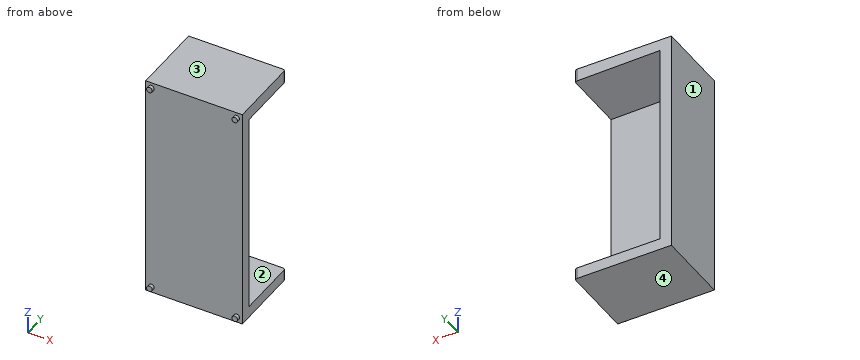
from build123d import *

# Parameters (mm, degrees)
BOSS_EXTRUDE1_DEPTH = 2000
CUT_EXTRUDE1_DEPTH  = 550
SKETCH4_R           = 25
BOSS_EXTRUDE2_DEPTH = 30


with BuildPart() as part:
    # Sketch1 → Boss-Extrude1 (new body)
    with BuildSketch(Plane.XY):
        with BuildLine():
            Line((-425, 270.9650644), (405, 270.9650644))
            ThreePointArc((405, 270.9650644), (419.142135624, 265.107200024), (425, 250.9650644))
            Line((425, 250.9650644), (425, -379.0349356))
            Line((425, -379.0349356), (-425, -379.0349356))
            Line((-425, -379.0349356), (-425, 270.9650644))
        make_face()
    extrude(amount=BOSS_EXTRUDE1_DEPTH)

    # Sketch3 → Cut-Extrude1 (cut)
    with BuildSketch(Plane(origin=(0, 270.9650644, 0), x_dir=(1, 0, 0), z_dir=(0, 1, 0))):
        Polygon((-325, -100), (425, -100), (425, -1887.575015641), (-325, -1900), align=None)
    extrude(amount=-CUT_EXTRUDE1_DEPTH, mode=Mode.SUBTRACT)

    # Sketch4 → Boss-Extrude2 (add)
    with BuildSketch(Plane(origin=(0, -379.0349356, 0), x_dir=(-1, 0, 0), z_dir=(0, -1, 0))):
        with Locations((375, -1950)):
            Circle(SKETCH4_R)
        with Locations((-375, -1950)):
            Circle(SKETCH4_R)
        with Locations((375, -50)):
            Circle(SKETCH4_R)
        with Locations((-375, -50)):
            Circle(SKETCH4_R)
    extrude(amount=BOSS_EXTRUDE2_DEPTH)


solid = part.part
Source: CAD feature listing. Evaluate the final solid. Frame: model axes, mm. Face numbers are marked on the shaded views. Round coordinates to 2 decimals unless told otherwise and drop trailing zeros. Loops run counter-clockwise (first coordinate to the right, second up) from the corner with the lowest first, then second, coordinate; pieces in that order, holes last. Notation, with made-up numbers: M 24,-18 L 42,-18 A28 ccw 42,5 Z; hole C 36.5,12 d3. An arc over 180 degrees is marked long. Return JSON: item names as keys, results as strings. Group by question number.
1. Material intervals for line 1 along Z through (x, y) = (-307.5, 115); line 2 along X through (y, z) = (50.5, 467.5); line 3 along Y through (x, z) = (-161.5, 659), sorted ascending. Write a range as from..to.
2. Pin query (flat end, axial travel): pin 1 (8 mm diameter, centred on x = 4, z = 1286.5, fed in from -Y); pin 2 (1 mm diameter, centred on x = 45, z = 1372.5, fed in from +Y); pin 3 (2 mm diameter, centred on y = -142.5, z = 251.5, fed in from +X). Return the tip coordinate at first contact, or that it passes through.
3. Section query C-C on x = -243.5. Output: boundary loops of the cut face in (y, z), and give its area (3 significant figures).
4. Section query B-B on y = 85. Output: boundary loops of the cut face in (x, z), and give its area (3 significant figures).
5. Section query A-A on z = 517. Output: boundary loops of the cut face in (x, y).
6. Mould query, pull axis Z, two halves, no side actions, for the marked faces 1, 2, 3 and 4. Classes: released by +Z, released by -Z, zero draft, split by the parting line, or undercut.
7. Section query D-D on z = 1950. Output: boundary loops of the cut face in (x, y), and give its area (3 significant figures).
Checks:
{
 "1": {"line 1": "z = 0..100, 1899.71..2000", "line 2": "x = -425..-325", "line 3": "y = -379.03..-279.03"},
 "2": {"pin 1": "stops at y = -379.03", "pin 2": "stops at y = -279.03", "pin 3": "stops at x = -325"},
 "3": {"outline": "M -379.03,0 L 270.97,0 L 270.97,100 L -279.03,100 L -279.03,1898.65 L 270.97,1898.65 L 270.97,2000 L -379.03,2000 Z", "area": "311,000 mm²"},
 "4": {"outline": "M -425,0 L 425,0 L 425,100 L -325,100 L -325,1900 L 425,1887.58 L 425,2000 L -425,2000 Z", "area": "355,000 mm²"},
 "5": {"outline": "M -425,-379.03 L 425,-379.03 L 425,-279.03 L -325,-279.03 L -325,270.97 L -425,270.97 Z"},
 "6": {"face 1": "zero draft", "face 2": "undercut", "face 3": "released by +Z", "face 4": "released by -Z"},
 "7": {"outline": "M -425,-379.03 L -400,-379.03 L -400,-409.03 L -350,-409.03 L -350,-379.03 L 350,-379.03 L 350,-409.03 L 400,-409.03 L 400,-379.03 L 425,-379.03 L 425,250.97 A20 ccw 405,270.97 L -425,270.97 Z", "area": "555,000 mm²"}
}
